Verification items for the finished model (mm, model axes). Face numbers are marked on the shaded views. A direction names the side the tool comes from. Round coordinates to 2 decimals unless told otherwise and drop trailing zeros. Order: outer loops, then holes, each group sorted by start corner. A loop starts at its lowest first (then second) coordinate and runs counter-clockwise, first axis right, second up. Notation, with made-up numbers: M 1,80 L 11,80 A15 cw 11,109 Z; hole C -7.75,-28.5 d5. An arc over 180 degrees is marked long. Answer as a JSON object with one key per item and string values. Group by question number.
```python
from build123d import *

# Parameters (mm, degrees)
F2_DEPTH      = 80
F1_W          = 5
F1_H          = 25
F3_DEPTH      = 80
F4_R          = 3.25
F5_DEPTH      = 25
F5_DEPTH_BACK = 25


with BuildPart() as f2:
    # F0 (on Top) → F2 (new body)
    with BuildSketch(Plane.XY):
        with BuildLine():
            Line((-12.5, -11.25), (12.5, -11.25))
            Line((12.5, -11.25), (12.5, 11.25))
            ThreePointArc((12.5, 11.25), (11.2575846496, 16.6829354732), (7.777313943, 21.0358769577))
            Line((7.777313943, 21.0358769577), (6.5329437122, 19.4701366445))
            ThreePointArc((6.5329437122, 19.4701366445), (9.4563711057, 15.8136657975), (10.5, 11.25))
            Line((10.5, 11.25), (10.5, -9.25))
            Line((10.5, -9.25), (-10.5, -9.25))
            Line((-10.5, -9.25), (-10.5, 11.25))
            ThreePointArc((-10.5, 11.25), (-9.4563711057, 15.8136657975), (-6.5329437122, 19.4701366445))
            Line((-6.5329437122, 19.4701366445), (-7.777313943, 21.0358769577))
            ThreePointArc((-7.777313943, 21.0358769577), (-11.2575846496, 16.6829354732), (-12.5, 11.25))
            Line((-12.5, 11.25), (-12.5, -11.25))
        make_face()
    extrude(amount=F2_DEPTH)

    # F1 (on Top) → F3 (join)
    with BuildSketch(Plane.XY):
        with Locations((0, -23.75)):
            Rectangle(F1_W, F1_H)
    extrude(amount=F3_DEPTH)

    # F4 (on Right) → F5 (cut, two sides)
    with BuildSketch(Plane.YZ) as f5_sk:
        with Locations((-23.75, 20)):
            Circle(F4_R)
        with Locations((-23.75, 60)):
            Circle(F4_R)
    extrude(amount=-F5_DEPTH, mode=Mode.SUBTRACT)
    extrude(f5_sk.sketch, amount=F5_DEPTH_BACK, mode=Mode.SUBTRACT)


solid = f2.part
```
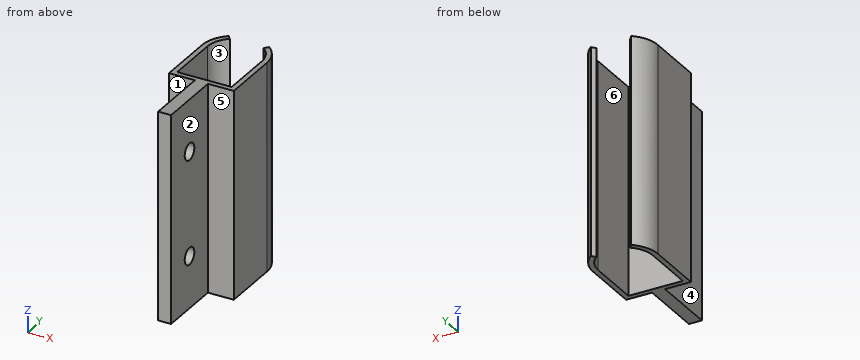
Q1. Gauge pin test, flat ends, axial feed: pin 1 Ø2 at (y, z) = (-13, 61) entering from +X; pin 2 Ø8 at (x, z) = (-10, 53.5) entering from -Y; pin 3 Ø1.5 at (x, z) = (-6, 11) entering from +Y. Record the tip position at first contact, or that the pin passes through.
Q2. Tool access check on the marked faces 4, 5 and 6. Record the directions out of +Z, -Z, +X, -X, +Y, -Y that give a thin tool (end or side, any length) a straight path to the whole face; none if there is none.
Q3. Cross-section at A-A, the plane y = -23.75. Record the cut outline in (x, z), then the cut area to 3 significant figures.
Q4. Thickness scan on line 1 (Z direction, x = -0.35, y = -23.75); line 2 (X direction, y = 7, z = 6.5); line 3 (Y direction, x = -0.35, z = 20). Record the ranges inside material, lowest first. Write a range as from..to.
Q5. Cross-section at C-C, the plane y = 10. Record the cut outline in (x, z).
Q6. Release check for a two-part mould opening along Y. For the marked faces 1, 2 and 3 record: released by +Y, released by -Y, zero draft, split by the parting line, or undercut.
Q7. Cross-section at D-D, the plane z = 49. Record the cut outline in (x, y), then the cut area to 3 significant figures.
Q8. Cross-section at B-B, the plane z = 20. Record the cut outline in (x, y), then the cut area to 3 significant figures.
Conclusion:
{
 "1": {"pin 1": "x = 2.5", "pin 2": "y = -11.25", "pin 3": "y = 19.74"},
 "2": {"face 4": "+Z, -Z, -X, -Y", "face 5": "+Z, -Z, +X, -Y", "face 6": "+Z, -Z"},
 "3": {"outline": "M -2.5,0 L 2.5,0 L 2.5,16.75 L -2.5,16.75 Z; M -2.5,23.25 L 2.5,23.25 L 2.5,56.75 L -2.5,56.75 Z; M -2.5,63.25 L 2.5,63.25 L 2.5,80 L -2.5,80 Z", "area": "335 mm2"},
 "4": {"line 1": "0..16.75, 23.25..56.75, 63.25..80", "line 2": "-12.5..-10.5, 10.5..12.5", "line 3": "-36.25..-27, -20.5..-9.25"},
 "5": {"outline": "M -12.5,0 L -10.5,0 L -10.5,80 L -12.5,80 Z; M 10.5,0 L 12.5,0 L 12.5,80 L 10.5,80 Z"},
 "6": {"face 1": "released by -Y", "face 2": "zero draft", "face 3": "undercut"},
 "7": {"outline": "M -12.5,-11.25 L -2.5,-11.25 L -2.5,-36.25 L 2.5,-36.25 L 2.5,-11.25 L 12.5,-11.25 L 12.5,11.25 A12.5 ccw 7.78,21.04 L 6.53,19.47 A10.5 cw 10.5,11.25 L 10.5,-9.25 L -10.5,-9.25 L -10.5,11.25 A10.5 cw -6.53,19.47 L -7.78,21.04 A12.5 ccw -12.5,11.25 Z", "area": "298 mm2"},
 "8": {"outline": "M -12.5,-11.25 L -2.5,-11.25 L -2.5,-20.5 L 2.5,-20.5 L 2.5,-11.25 L 12.5,-11.25 L 12.5,11.25 A12.5 ccw 7.78,21.04 L 6.53,19.47 A10.5 cw 10.5,11.25 L 10.5,-9.25 L -10.5,-9.25 L -10.5,11.25 A10.5 cw -6.53,19.47 L -7.78,21.04 A12.5 ccw -12.5,11.25 Z; M -2.5,-36.25 L 2.5,-36.25 L 2.5,-27 L -2.5,-27 Z", "area": "266 mm2"}
}
